Autodesk Inventor part; units mm, degrees
ref_plane "YZ Plane" through (0, 0, 0) normal (1, 0, 0) x (0, 1, 0)
ref_plane "XZ Plane" through (0, 0, 0) normal (0, 1, 0) x (-1, 0, 0)
ref_plane "XY Plane" through (0, 0, 0) normal (0, 0, 1) x (1, 0, 0)
sketch "Sketch1" plane through (0, 0, 0) normal (0, 1, 0) x (-1, 0, 0)
  circle A0 centre (0, 0) radius 8 construction
  circle A1 centre (0, -8) radius 1.5
  circle A2 centre (6.9282, -4) radius 1.5
  circle A3 centre (6.9282, 4) radius 1.5
  circle A4 centre (0, 8) radius 1.5
  circle A5 centre (-6.9282, 4) radius 1.5
  circle A6 centre (-6.9282, -4) radius 1.5
  circle A7 centre (0, 0) radius 5
  line L0 (12.7, 19.05) -> (-12.7, 19.05)
  line L1 (-12.7, 19.05) -> (-12.7, -19.05)
  line L2 (-12.7, -19.05) -> (12.7, -19.05)
  line L3 (12.7, -19.05) -> (12.7, 19.05)
  line L4 (12.7, 19.05) -> (-12.7, -19.05) construction
  line L5 (-12.7, 19.05) -> (12.7, -19.05) construction
  dimension "d0" = 16
  dimension "d1" = 3
  dimension "d4" = 360
  dimension "d6" = 10
  dimension "d7" = 25.4
  dimension "d8" = 38.1
extrude "Extrusion1" add sketch "Sketch1" along normal blind 6.35
properties part number "rev holes"
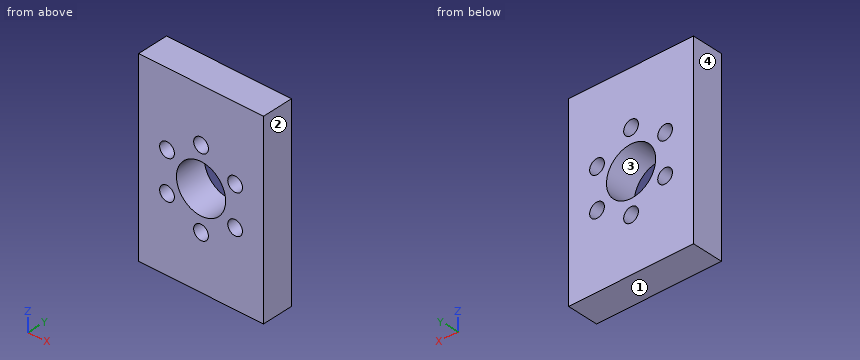
Can you work these out from the model? Positions are in its coordinate system, mm. Face numbers are marked on the shaded views. Give positions to 0.01 mm unless a question says otherwise; leave off trailing zeros. Write each loop counter-clockwise with the first axis right and the second up, starting at its lowest first coordinate (ties: lowest second). Pieces come first, ordered by that corner, then holes. Notation, with made-up numbers: M 64.5,-9 L 121.5,-9 A26 ccw 121.5,12 Z; hole C 25.5,86.5 d5. An arc over 180 degrees is marked long. Answer in a Markdown table with one row per item. Add a question column.
Item 1: Imagine slicing it at A-A, the plane x = 0. Write out the boundary of the cut face in (y, z).
Item 2: Imagine slicing it at C-C, the plane y = 3.25. Write out the boundary of the cut face in (x, z), plus the area to 3 significant figures.
Item 3: We'd pull the mould along X, two halves only. Please class the marked faces 1, 2, 3 and 4: released by +X, released by -X, zero draft, split by the parting line, or undercut.
Item 4: Imagine slicing it at B-B, the plane z = 0. Write out the boundary of the cut face in (x, y), plus the area to 3 significant figures.
Item 5: Please list where these lines run through material, in increasing order: L1, parallel to Z at x = 0, y = 2.25; L2, parallel to Z at x = -7, y = 2.25; L3, parallel to X at y = 2.5, z = 4.5.
Item 6: Imagine slicing it at D-D, the plane z = -4. Write out the boundary of the cut face in (x, y).
Evaluation:
| question | item | result |
|---|---|---|
| 1 | outline | M 0,-19.05 L 6.35,-19.05 L 6.35,-9.5 L 0,-9.5 Z; M 0,-6.5 L 6.35,-6.5 L 6.35,-5 L 0,-5 Z; M 0,5 L 6.35,5 L 6.35,6.5 L 0,6.5 Z; M 0,9.5 L 6.35,9.5 L 6.35,19.05 L 0,19.05 Z |
| 2 | outline | M -12.7,-19.05 L 12.7,-19.05 L 12.7,19.05 L -12.7,19.05 Z; hole C -6.93,-4 d3; hole C -6.93,4 d3; hole C 0,0 d10; hole C 0,-8 d3; hole C 0,8 d3; hole C 6.93,-4 d3; hole C 6.93,4 d3 |
| 2 | area | 847 mm² |
| 3 | face 1 | zero draft |
| 3 | face 2 | released by +X |
| 3 | face 3 | undercut |
| 3 | face 4 | released by -X |
| 4 | outline | M -12.7,0 L -5,0 L -5,6.35 L -12.7,6.35 Z; M 5,0 L 12.7,0 L 12.7,6.35 L 5,6.35 Z |
| 4 | area | 97.8 mm² |
| 5 | L1 | z = -19.05 to -9.5, -6.5 to -5, 5 to 6.5, 9.5 to 19.05 |
| 5 | L2 | z = -19.05 to -5.5, -2.5 to 2.5, 5.5 to 19.05 |
| 5 | L3 | x = -12.7 to -8.34, -5.51 to -2.18, 2.18 to 5.51, 8.34 to 12.7 |
| 6 | outline | M -12.7,0 L -8.43,0 L -8.43,6.35 L -12.7,6.35 Z; M -5.43,0 L -3,0 L -3,6.35 L -5.43,6.35 Z; M 3,0 L 5.43,0 L 5.43,6.35 L 3,6.35 Z; M 8.43,0 L 12.7,0 L 12.7,6.35 L 8.43,6.35 Z |
